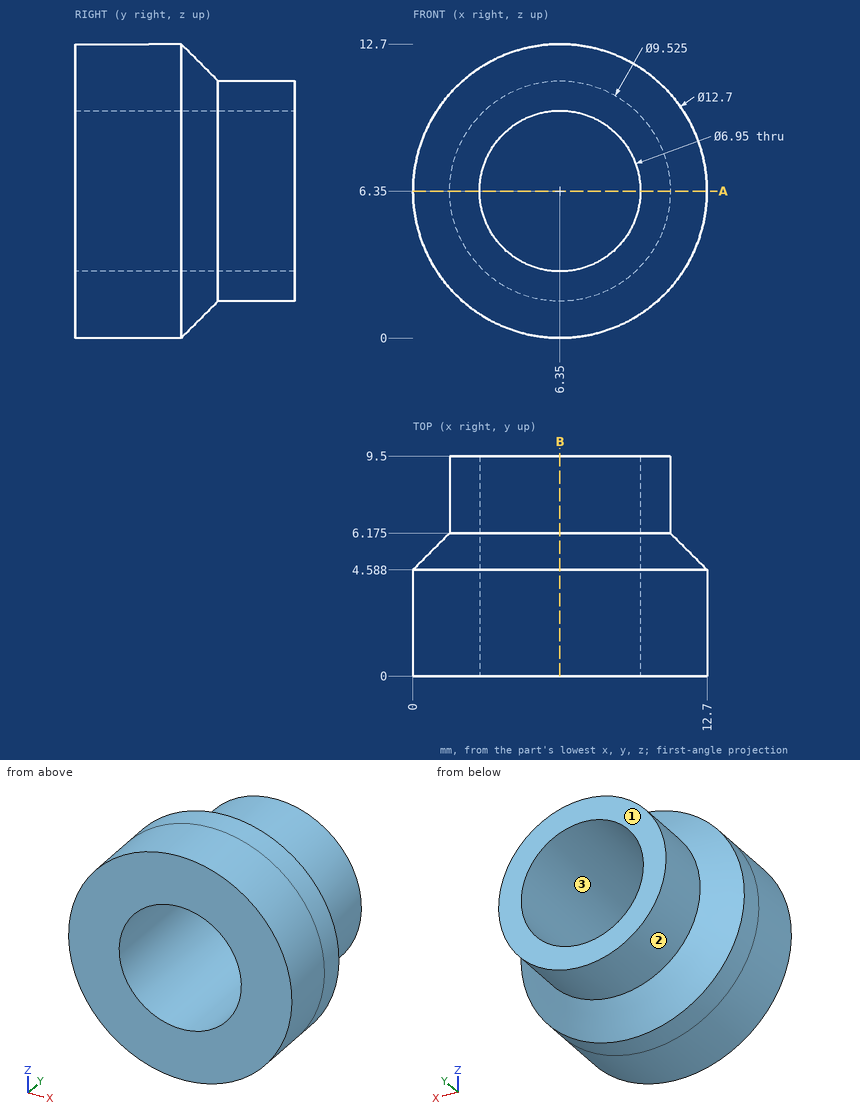
Drawing for the job (mm, zero at the part's lowest x, y, z). Give positions to 0.01 mm unless a question says otherwise; leave off trailing zeros. Loops run counter-clockwise (first coordinate to the right, second up) from the corner with the lowest first, then second, coordinate; pieces in that order, holes last.
1) Band-saw the part on A-A on z = 6.35. List the corners of the cut face in (x, y) (1 decimal).
Values follow:
outline: (0, 0) - (2.9, 0) - (2.9, 9.5) - (1.6, 9.5) - (1.6, 6.2) - (0, 4.6) - close; (9.8, 0) - (12.7, 0) - (12.7, 4.6) - (11.1, 6.2) - (11.1, 9.5) - (9.8, 9.5) - close
2) Two-plate mould, pull along X, no slides. Class the marked faces 1, 2 and 3: released by +X, released by -X, zero draft, split by the parting line, or undercut.
Values follow:
face 1: zero draft
face 2: split by the parting line
face 3: undercut
3) Band-saw the part on B-B on x = 6.35. List the corners of the cut face in (y, z) (1 decimal).
Values follow:
outline: (0, 0) - (4.6, 0) - (6.2, 1.6) - (9.5, 1.6) - (9.5, 2.9) - (0, 2.9) - close; (0, 9.8) - (9.5, 9.8) - (9.5, 11.1) - (6.2, 11.1) - (4.6, 12.7) - (0, 12.7) - close
4) Drop flat-ended pins along their axis: P1, Ø3, axis at x = 1.5, y = 5.5, coming from the -Z side; P2, Ø3, axis at x = 3.5, z = 9, coming from the -Y side; P3, Ø2, axis at y = 1.5, z = 9, coming from the -X side; P4, Ø2, axis at x = 1.5, y = 1, coming from the -Z side. Give the stop position or say it passes through.
Values follow:
P1: stops at z = 1.16
P2: stops at y = 0
P3: stops at x = 0.22
P4: stops at z = 1.3
5) Probe line 1 along X through (y, z) = (3.5, 6.35) (1 decimal); line 2 along Z through (x, y) = (6.25, 4.5); line 3 along X through (y, z) = (7.5, 6.35) (1 decimal). List the from-to ranges inside material, lowest first.
Values follow:
line 1: x = 0 to 2.9, 9.8 to 12.7
line 2: z = 0 to 2.88, 9.82 to 12.7
line 3: x = 1.6 to 2.9, 9.8 to 11.1
